Read the model definition and answer for the solid it produces. Units are mm, in the model's axes. Face numbers are marked on the shaded views. Coordinates: 2 decimals unless noted, no trailing zeros. Write each loop counter-clockwise with the first axis right and the second up, starting at its lowest first coordinate (ties: lowest second). Pieces come first, ordered by that corner, then holes. Notation, with made-up numbers: M -3,-35 L 28,-35 A18 ccw 28,-7 Z; hole C -1,88 d2. An arc over 180 degrees is marked long. Use a Markdown table: item, result. Add a question column.
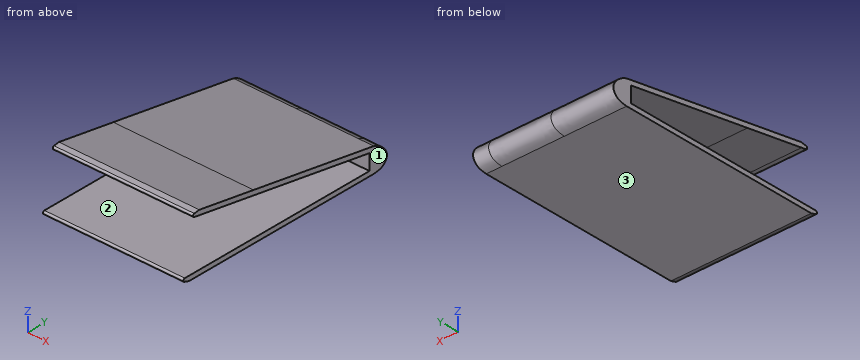
from build123d import *

# Parameters (mm, degrees)
F1_DEPTH = 20
F2_DEPTH = 25
F3_R     = 0.5


with BuildPart() as f1:
    # F0 (on Right) → F1 (new body, symmetric)
    with BuildSketch(Plane.YZ):
        with BuildLine():
            Line((-41, 12), (0, 5))
            Line((0, 5), (0, 0))
            Line((0, 0), (-13, 0))
            Line((-13, 0), (-60, 0))
            Line((-60, 0), (-68.1802767269, 0))
            Line((-68.1802767269, 0), (-63.4105807199, -1.5))
            Line((-63.4105807199, -1.5), (-15.9391719951, -1.5))
            Line((-15.9391719951, -1.5), (1.5, -1.5))
            add(Edge.make_bspline(
                [(1.5, 6.265607391), (3.9644898677, 5.4991167031), (6.8949081715, 2.4881725012), (5.5893039586, -0.1081592765), (4.0791571197, -1.2143747147), (2.4017938603, -1.4076838823), (1.5, -1.5)],
                knots=[0, 0, 0, 0, 0.3589021343, 0.5755750332, 0.7680765927, 1, 1, 1, 1], degree=3))
            Line((1.5, 6.265607391), (-40.7475553057, 13.4786046383))
            Line((-40.7475553057, 13.4786046383), (-59.8354584084, 16.7375149241))
            Line((-59.8354584084, 16.7375149241), (-64.7895661956, 16.0616332529))
            Line((-64.7895661956, 16.0616332529), (-60, 15.243902439))
            Line((-60, 15.243902439), (-41, 12))
        make_face()
    extrude(amount=F1_DEPTH, both=True)

    # F0 (on Right) → F2 (join)
    with BuildSketch(Plane.YZ):
        with BuildLine():
            Line((-41, 12), (0, 5))
            Line((0, 5), (0, 0))
            Line((0, 0), (-13, 0))
            Line((-13, 0), (-60, 0))
            Line((-60, 0), (-68.1802767269, 0))
            Line((-68.1802767269, 0), (-63.4105807199, -1.5))
            Line((-63.4105807199, -1.5), (-15.9391719951, -1.5))
            Line((-15.9391719951, -1.5), (1.5, -1.5))
            add(Edge.make_bspline(
                [(1.5, 6.265607391), (3.9644898677, 5.4991167031), (6.8949081715, 2.4881725012), (5.5893039586, -0.1081592765), (4.0791571197, -1.2143747147), (2.4017938603, -1.4076838823), (1.5, -1.5)],
                knots=[0, 0, 0, 0, 0.3589021343, 0.5755750332, 0.7680765927, 1, 1, 1, 1], degree=3))
            Line((1.5, 6.265607391), (-40.7475553057, 13.4786046383))
            Line((-40.7475553057, 13.4786046383), (-59.8354584084, 16.7375149241))
            Line((-59.8354584084, 16.7375149241), (-64.7895661956, 16.0616332529))
            Line((-64.7895661956, 16.0616332529), (-60, 15.243902439))
            Line((-60, 15.243902439), (-41, 12))
        make_face()
    extrude(amount=F2_DEPTH)

    # F3
    f3_edges = [f1.edges().sort_by_distance(p)[0] for p in [
        (2.5, -64.789566, 16.061633),
        (2.5, -68.180277, 0),
    ]]
    fillet(f3_edges, radius=F3_R)


solid = f1.part
Item 1: Determine the mould class of the marked faces 1, 2 and 3 for opening direction Z: pulls with the +Z half, pulls with the -Z half, needs draft (parallel to the pull), parting line crosses it, or undercut.
Item 2: Each of these flat-tipped pins is pushed along its axis until it touches: pin 1 (2 mm diameter, centred on y = -35, z = 2, fed in from +X); pin 2 (4 mm diameter, centred on x = -5.5, z = 2.5, fed in from -Y); pin 3 (13.5 mm diameter, centred on x = 3, y = -42, fed in from +Z). Where does it stop, or does it pass through?
Item 3: Find section B-B on z = 11.25. Give the vertices of the cut face in (x, y), then the cut area to 3 significant figures.
Item 4: Find section A-A on y = -56. Give the vertices of the cut face in (x, z), then the cut area to 3 significant figures.
Item 5: Consider probe 1 along Z at (x, y) = (-8.5, -40); probe 2 along Z at (x, y) = (3, -51.5); probe 3 along Y at (x, z) = (-15, 0.25). Determine where each line is inside the solid, lowest interval first.
Geometry says:
| question | item | result |
|---|---|---|
| 1 | face 1 | needs draft |
| 1 | face 2 | undercut |
| 1 | face 3 | pulls with the -Z half |
| 2 | pin 1 | passes through |
| 2 | pin 2 | stops at y = 0 |
| 2 | pin 3 | stops at z = 14.84 |
| 3 | outline | M -20,-36.61 L 25,-36.61 L 25,-27.69 L -20,-27.69 Z |
| 3 | area | 401 mm2 |
| 4 | outline | M -20,-1.5 L 25,-1.5 L 25,0 L -20,0 Z; M -20,14.56 L 25,14.56 L 25,16.08 L -20,16.08 Z |
| 4 | area | 136 mm2 |
| 5 | probe 1 | z = -1.5 to 0, 11.83 to 13.35 |
| 5 | probe 2 | z = -1.5 to 0, 13.79 to 15.31 |
| 5 | probe 3 | y = 0 to 5.66 |
